```python
from build123d import *

# Parameters (mm, degrees)
BOX053_W                  = 10
BOX053_H                  = 4
BOX053_DEPTH              = 5.8
CYLINDER066_R             = 2.2
CYLINDER066_DEPTH         = 20
CYLINDER067_R             = 2.2
CYLINDER067_DEPTH         = 20
CYLINDER064_R             = 5
CYLINDER064_DEPTH         = 16
BOX051_W                  = 30
BOX051_H                  = 8
BOX051_DEPTH              = 16
FUSION036_PITCH_ANGLE     = 90
FUSION036_PLACEMENT_ANGLE = 90


with BuildPart() as quader032:
    # Box053 → Box053 (new body)
    with BuildSketch(Plane(origin=(-5, 8, 5), x_dir=(1, 0, 0), z_dir=(0, 0, 1))):
        with Locations((5, 2)):
            Rectangle(BOX053_W, BOX053_H)
    extrude(amount=BOX053_DEPTH)


with BuildPart() as zylinder055:
    # Cylinder066 → Cylinder066 (new body)
    with BuildSketch(Plane(origin=(-10, 9, 8), x_dir=(1, 0, 0), z_dir=(0, -1, 0))):
        Circle(CYLINDER066_R)
    extrude(amount=CYLINDER066_DEPTH)


with BuildPart() as zylinder056:
    # Cylinder067 → Cylinder067 (new body)
    with BuildSketch(Plane(origin=(10, 9, 8), x_dir=(1, 0, 0), z_dir=(0, -1, 0))):
        Circle(CYLINDER067_R)
    extrude(amount=CYLINDER067_DEPTH)


with BuildPart() as zylinder053:
    # Cylinder064 → Cylinder064 (new body)
    with BuildSketch(Plane.XY):
        Circle(CYLINDER064_R)
    extrude(amount=CYLINDER064_DEPTH)


with BuildPart() as y_mount_bottom:
    # Box051 → Box051 (new body)
    with BuildSketch(Plane(origin=(-15, 0, 0), x_dir=(1, 0, 0), z_dir=(0, 0, 1))):
        with Locations((15, 4)):
            Rectangle(BOX051_W, BOX051_H)
    extrude(amount=BOX051_DEPTH)

    # Cut071: cut Zylinder053
    add(zylinder053.part, mode=Mode.SUBTRACT)

    # Cut073: cut Zylinder056
    add(zylinder056.part, mode=Mode.SUBTRACT)

    # Cut074: cut Zylinder055
    add(zylinder055.part, mode=Mode.SUBTRACT)

    # Fusion036: union Quader032
    add(quader032.part)


with BuildPart() as y_mount_bottom_1:
    # Fusion036 pitch: moved
    add(y_mount_bottom.part.rotate(Axis((0, 0, 0), (0, 1, 0)), FUSION036_PITCH_ANGLE))


with BuildPart() as y_mount_bottom_2:
    # Fusion036 placement: moved
    add(y_mount_bottom_1.part.moved(Location((-9.75, -14.15, 29.85))).rotate(Axis((-9.75, -14.15, 29.85), (0, 0, 1)), FUSION036_PLACEMENT_ANGLE))


solid = y_mount_bottom_2.part
```
CAD build for the part. Positions are in the model's coordinates, mm. A direction names the side the tool comes from. Coordinates: 2 decimals unless noted, no trailing zeros. Write each loop counter-clockwise with the first axis right and the second up, starting at its lowest first coordinate (ties: lowest second). Pieces come first, ordered by that corner, then holes. Notation, with made-up numbers: (-26, 21.25) -> (-5, 21.25) arc R11 ccw to (-5, 33.25) -> close; hole circle Ø4 at (-28.5, 56.25). An arc over 180 degrees is marked (long way). Use CSV: the item, a comma, the result in double quotes. Start each with the question number.
Item 1: Two-plate mould, pull along Z, no slides. Class faces 1 (the cylindrical face through (-13.806, -4.295, 38.667)), 2 (the flat face through (-16, -14.15, 30)), 3 (the flat face through (-20, -6, 24.85)): +Z half, -Z half, draft (parallel to the pull), parting line (faces both ways), or undercut.
Item 2: Drop flat-ended pins along their axis: P1, Ø3, axis at x = -20.5, y = -6, coming from the +Z side; P2, Ø3, axis at x = -20, z = 28, coming from the -Y side; P3, Ø5, axis at y = -6.15, z = 19.85, coming from the -X side; P4, Ø2.5, axis at y = -6.15, z = 39.85, coming from the -X side. Give the stop position or say it passes through.
Item 3: Tool access for faces 4 (the flat face through (-21.75, -6, 30)), 5 (the flat face through (-20, -9.15, 30)), 6 (the flat face through (-20, -6, 34.85)), 7 (the flat face through (-9.75, -8, 42)), 8 (the flat face through (-20, -3.35, 30)): list every direction of +Z, -Z, +X, -X, +Y, -Y with a clear straight run to the whole face (end or side of a thin tool).
Item 4: Band-saw the part on B-B, the plane z = 39.85. Write the cut outline in (x, y), plus the area to 3 significant figures.
Item 5: Band-saw the part on A-A, the plane x = -12.75. Write the cut outline in (y, z), plus the area to 3 significant figures.
Item 6: Band-saw the part on C-C, the plane y = -8.75. Write the cut outline in (x, z), plus the area to 3 significant figures.
Item 7: Wall check: probe 1 along Y at (x, z) = (-16, 19.85); probe 2 along Z at (x, y) = (-17.5, -7.75); probe 3 along Z at (x, y) = (-10.25, -5). Give the ranges that are in metal, low to high.
Item 8: Band-saw the part on D-D, the plane z = 29.85. Write the cut outline in (x, y), plus the area to 3 significant figures.
Response values:
1,face 1,"undercut"
1,face 2,"draft"
1,face 3,"-Z half"
2,P1,"stops at z = 34.85"
2,P2,"stops at y = -9.15"
2,P3,"stops at x = -17.75"
2,P4,"passes through"
3,face 4,"+Z, -Z, -X, +Y, -Y"
3,face 5,"+Z, -Z, -X, -Y"
3,face 6,"+Z, -X, +Y, -Y"
3,face 7,"+Z, -Z, +X, +Y, -Y"
3,face 8,"+Z, -Z, -X, +Y"
4,outline,"(-17.75, -14.15) -> (-9.75, -14.15) -> (-9.75, -8.35) -> (-17.75, -8.35) -> close; (-17.75, -3.95) -> (-9.75, -3.95) -> (-9.75, 1.85) -> (-17.75, 1.85) -> close"
4,area,"92.8 mm2"
5,outline,"(-14.15, 14.85) -> (1.85, 14.85) -> (1.85, 25.85) -> (-14.15, 25.85) -> close; (-14.15, 33.85) -> (1.85, 33.85) -> (1.85, 44.85) -> (-14.15, 44.85) -> close; hole circle Ø4.4 at (-6.15, 19.85); hole circle Ø4.4 at (-6.15, 39.85)"
5,area,"322 mm2"
6,outline,"(-21.75, 24.85) -> (-17.75, 24.85) -> (-17.75, 14.85) -> (-9.75, 14.85) -> (-9.75, 24.85) arc R5 cw to (-9.75, 34.85) -> (-9.75, 44.85) -> (-17.75, 44.85) -> (-17.75, 34.85) -> (-21.75, 34.85) -> close"
6,area,"241 mm2"
7,probe 1,"y = -14.15 to -8.35, -3.95 to 1.85"
7,probe 2,"z = 14.85 to 18.34, 21.36 to 38.34, 41.36 to 44.85"
7,probe 3,"z = 14.85 to 17.97, 21.73 to 24.88, 34.82 to 37.97, 41.73 to 44.85"
8,outline,"(-21.75, -9.15) -> (-17.75, -9.15) -> (-17.75, -14.15) -> (-14.75, -14.15) -> (-14.75, 1.85) -> (-17.75, 1.85) -> (-17.75, -3.35) -> (-21.75, -3.35) -> close"
8,area,"71.2 mm2"
